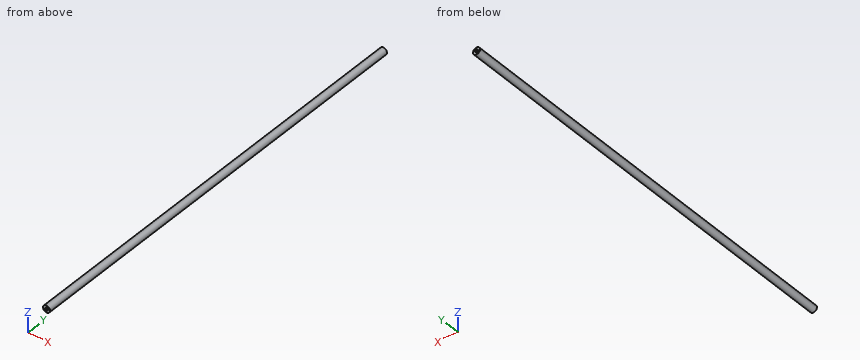
from build123d import *

# Parameters (mm, degrees)
SKETCH3_R               = 7.5
BOSS_EXTRUDE1_DEPTH     = 900
SHELL2_T                = 2
SKETCH4_R               = 3
CUT_EXTRUDE1_DEPTH      = 1
CUT_EXTRUDE1_DEPTH_BACK = 901


with BuildPart() as part:
    # Sketch3 → Boss-Extrude1 (new body)
    with BuildSketch(Plane(origin=(0, 0, 0), x_dir=(1, 0, 0), z_dir=(0, 1, 0))):
        Circle(SKETCH3_R)
    extrude(amount=BOSS_EXTRUDE1_DEPTH)

    # Shell2 (no face opened: a closed hollow body)
    add(offset(amount=-SHELL2_T, mode=Mode.PRIVATE), mode=Mode.SUBTRACT)

    # Sketch4 → Cut-Extrude1 (cut, two sides)
    with BuildSketch(Plane(origin=(0, 900, 0), x_dir=(1, 0, 0), z_dir=(0, 1, 0))) as cut_extrude1_sk:
        Circle(SKETCH4_R)
    extrude(amount=CUT_EXTRUDE1_DEPTH, mode=Mode.SUBTRACT)
    extrude(cut_extrude1_sk.sketch, amount=-CUT_EXTRUDE1_DEPTH_BACK, mode=Mode.SUBTRACT)


solid = part.part
For this review, take the finished solid that the model builds, in its own axes (mm). Round coordinates to 2 decimals unless told otherwise and drop trailing zeros. Write each loop counter-clockwise with the first axis right and the second up, starting at its lowest first coordinate (ties: lowest second). Pieces come first, ordered by that corner, then holes. Notation, with made-up numbers: (0, 29) -> (46, 29) arc R12 cw to (46, 37) -> close; hole circle Ø10 at (9.25, -23.75). An arc over 180 degrees is marked (long way). Use CSV: the item, a comma, the result in double quotes.
(1) Clearance check with flat-ended pins moving along their axes: P1, Ø4, axis at x = 3.5, y = 289.5, coming from the +Z side; P2, Ø1, axis at y = 380.5, z = -5, coming from the -X side; P3, Ø6, axis at x = 4, y = 319.5, coming from the -Z side. State where each tip first meets the part, or that it passes through.
Computed values:
P1,"z = 7.35"
P2,"x = -6"
P3,"z = -7.43"
(2) To check wall thickness, follow L1, parallel to Z at x = 0, y = 898.85; L2, parallel to Y at x = -4.5, z = -0.75. State the ranges of each line that lie inside material, in increasing order. Write a range as [from, to].
Computed values:
L1,"[-7.5, -3], [3, 7.5]"
L2,"[0, 2], [898, 900]"
(3) Consider section C-C, the plane y = 341.5. Give the boundary of the cut face in (x, z), plus the area to 3 significant figures.
Computed values:
outline,"circle Ø15 at (0, 0); hole circle Ø11 at (0, 0)"
area,"81.7 mm²"
(4) Consider section B-B, the plane z = 0. Give the boundary of the cut face in (x, y).
Computed values:
outline,"(-7.5, 0) -> (-3, 0) -> (-3, 2) -> (-5.5, 2) -> (-5.5, 898) -> (-3, 898) -> (-3, 900) -> (-7.5, 900) -> close; (3, 0) -> (7.5, 0) -> (7.5, 900) -> (3, 900) -> (3, 898) -> (5.5, 898) -> (5.5, 2) -> (3, 2) -> close"
(5) Consider section A-A, the plane x = 0. Give the boundary of the cut face in (y, z).
Computed values:
outline,"(0, -7.5) -> (900, -7.5) -> (900, -3) -> (898, -3) -> (898, -5.5) -> (2, -5.5) -> (2, -3) -> (0, -3) -> close; (0, 3) -> (2, 3) -> (2, 5.5) -> (898, 5.5) -> (898, 3) -> (900, 3) -> (900, 7.5) -> (0, 7.5) -> close"
